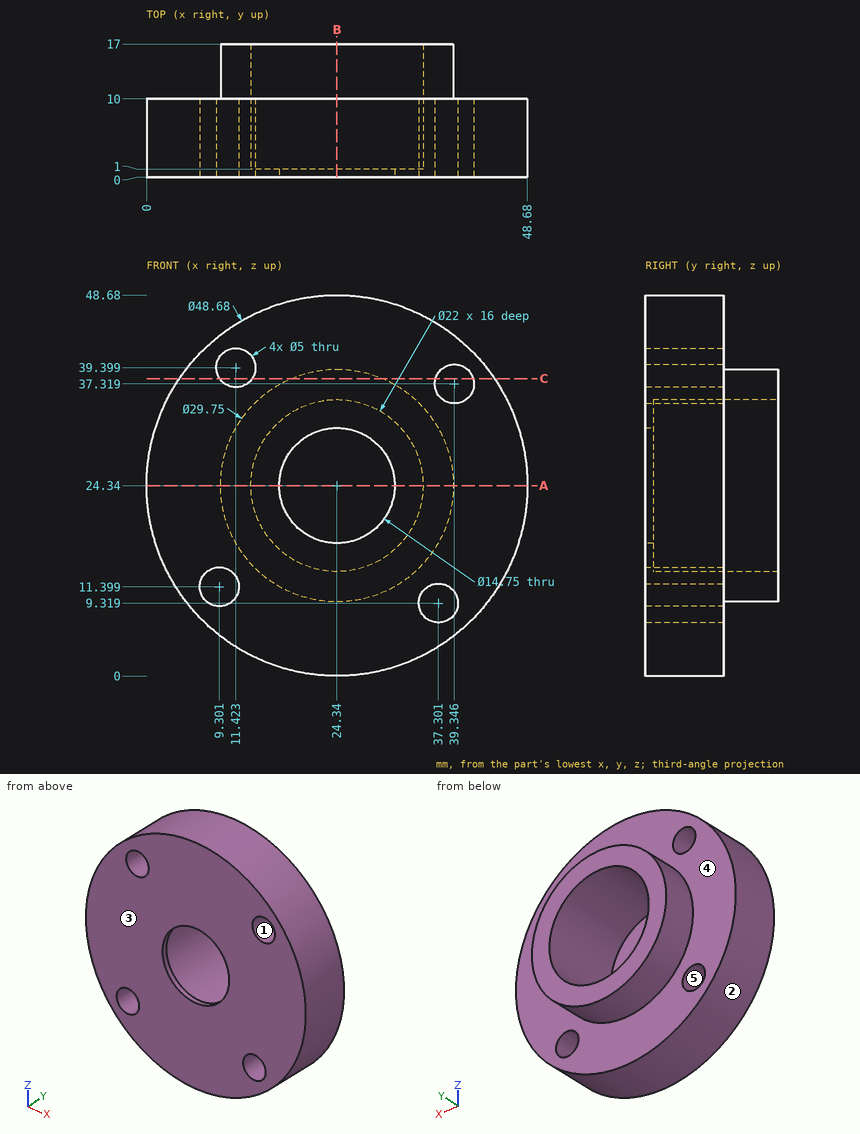
The figure shows three views and two pictorial views of one solid part (mm, origin at its lowest corner). Answer the questions. A direction names the side the tool comes from. Give positions to 0.01 mm unless a question says otherwise; leave off trailing zeros. Loops run counter-clockwise (first coordinate to the right, second up) from the corner with the lowest first, then second, coordinate; pieces in that order, holes last. Notation, with made-up numbers: M -30.75,83.25 L -9.75,83.25 A10 ccw -9.75,97.25 Z; hole C 65.5,-28 d8. An arc over 180 degrees is marked long. Write each question's results on one line, items separated by ' | '.
1. A tool of negligible diameter and unlimited length cuts with its end or side. For the marked faces 4 and 5, from which of +Z, -Z, +X, -X, +Y, -Y can it reach the whole face along a straight path? Write none if from no direction.
Values:
face 4: +Y | face 5: +Y, -Y
2. Section C-C on z = 38 is taken. Give the vertices of the cut face in (x, y) (1 decimal), plus the area to 3 significant figures.
Values:
outline: M 4.2,0 L 9.4,0 L 9.4,10 L 4.2,10 Z; M 13.5,0 L 36.9,0 L 36.9,10 L 30.2,10 L 30.2,17 L 18.5,17 L 18.5,10 L 13.5,10 Z; M 41.8,0 L 44.5,0 L 44.5,10 L 41.8,10 Z | area: 396 mm^2
3. Section A-A on z = 24.34 is taken. Give the vertices of the cut face in (x, y) (1 decimal).
Values:
outline: M 0,0 L 17,0 L 17,1 L 13.3,1 L 13.3,17 L 9.5,17 L 9.5,10 L 0,10 Z; M 31.7,0 L 48.7,0 L 48.7,10 L 39.2,10 L 39.2,17 L 35.3,17 L 35.3,1 L 31.7,1 Z
4. Given pin 1 (5 mm diameter, centred on x = 16.5, y = 7.5, fed in from +Z); pin 2 (8 mm diameter, centred on x = 9.3, z = 11.4, fed in from +Y); pin 3 (8 mm diameter, centred on x = 17.5, y = 11.5, fed in from -Z), each flat-ended and moving along its own axis, determine where each tip first touches the part or whether it passes through.
Values:
pin 1: stops at z = 48.09 | pin 2: stops at y = 10 | pin 3: stops at z = 0.2
5. The mould has two halves that part along X. Classify the marked faces 1, 2 and 3: pulls with the +X half, pulls with the -X half, needs draft (parallel to the pull), parting line crosses it, or undercut.
Values:
face 1: undercut | face 2: parting line crosses it | face 3: needs draft
6. Straight lines are drawn through the part: line 1 (X direction, y = 13.75, z = 24.34) (1 decimal); line 2 (Z direction, x = 11, y = 9.75) (1 decimal); line 3 (Y direction, x = 45, z = 26). For each, find the intervals that lie inside material, in ascending order. Write a range as [from, to].
Values:
line 1: x = [9.5, 13.3], [35.3, 39.2] | line 2: z = [4, 9.6], [13.2, 36.9], [41.9, 44.7] | line 3: y = [0, 10]
7. Section B-B on x = 24.34 is taken. Give the vertices of the cut face in (y, z) (1 decimal), plus the area to 3 significant figures.
Values:
outline: M 0,0 L 10,0 L 10,9.5 L 17,9.5 L 17,13.3 L 1,13.3 L 1,17 L 0,17 Z; M 0,31.7 L 1,31.7 L 1,35.3 L 17,35.3 L 17,39.2 L 10,39.2 L 10,48.7 L 0,48.7 Z | area: 328 mm^2
